Read the model definition and answer for the solid it produces. Units are mm, in the model's axes. A direction names the side the tool comes from. Round coordinates to 2 decimals unless told otherwise and drop trailing zeros. Order: outer loops, then holes, each group sorted by start corner. A loop starts at its lowest first (then second) coordinate and runs counter-clockwise, first axis right, second up. Notation, with made-up numbers: (79, 66) - (91, 66) arc R27 cw to (91, 97) - close; hole circle Ø7 at (47.25, -9.5). An arc over 180 degrees is marked (long way). One line per question, with ' | ' between items. Start each with the question number.
1) For faces 4 (the flat face through (-39, 2, -10)), 5 (the flat face through (44.24, 1.97, 3.73)), determine the directions among +Z, -Z, +X, -X, +Y, -Y from which every point of the face is accessible in a straight line to the end or side of a thin tool.
2) The mould has two halves that part along X. Classify faces 1 (the cylindrical face through (63.733, 1.972, -11.102)), 2 (the flat face through (20, 2, 0)), 3 (the flat face through (1, 2, -14)): pulls with the +X half, pulls with the -X half, needs draft (parallel to the pull), parting line crosses it, or undercut.
3) The part is cut by section A-A, the plane y = 1.4. Count the separate pieces of the cut face and the enclosed holes in it, plus the area to 3 significant figures.
4) Flat-ended cylindrical pins translate along their axes: pin 1 (2 mm diameter, centred on x = -59.47, z = -10, fed in from +Y); pin 2 (2 mm diameter, centred on x = 43, y = 1.5, fed in from +Z); pin 3 (1.5 mm diameter, centred on y = 1, z = -4, fed in from -X). Find the tip coordinate at first contact, or state that the pin passes through.
5) Straight lines are drawn through the part: line 1 (Z direction, x = -4.5, y = 3.45); line 2 (X direction, y = 2.9, z = -8.5); line 3 (X direction, y = 2.75, z = 2). For each, find the intervals that lie inside material, in ascending order. Write a range as from..to.
6) The part is cut by section C-C, the plane z = -0.5. Give the vertices of the cut face in (x, y).
7) The part is cut by section B-B, the plane x = -38. Give the vertices of the cut face in (y, z).
from build123d import *

# Parameters (mm, degrees)
SKETCH_1_R          = 1.5
SKETCH_1_W          = 40
SKETCH_1_H          = 20
EXTRUDE_1_DEPTH     = 4
FILLET_1_R          = 3
FILLET_2_R          = 3
SKETCH_2_R          = 1.75
CUT_EXTRUDE_1_DEPTH = 67.130086355


with BuildPart() as part:
    # 草图1 → 凸台-拉伸1 (new body)
    with BuildSketch(Plane(origin=(0, 0, 0), x_dir=(1, 0, 0), z_dir=(0, 1, 0))):
        with BuildLine():
            Line((-27, -14), (27, -14))
            Line((27, -14), (61.972111671, 6.837249964))
            ThreePointArc((61.972111671, 6.837249964), (63.714640377, 11.169883003), (60, 14))
            Line((60, 14), (27, 14))
            Line((27, 14), (-27, 14))
            Line((-27, 14), (-60, 14))
            ThreePointArc((-60, 14), (-63.714640377, 11.169883003), (-61.972111671, 6.837249964))
            Line((-61.972111671, 6.837249964), (-27, -14))
        make_face()
        with Locations(Location((-23.680960464, 5.529497849, 0), (0, 0, 270))):
            Circle(SKETCH_1_R, mode=Mode.SUBTRACT)
        with Locations(Location((-23.680960464, -5.529497849, 0), (0, 0, 90))):
            Circle(SKETCH_1_R, mode=Mode.SUBTRACT)
        with Locations(Location((23.680960464, -5.529497849, 0), (0, 0, 270))):
            Circle(SKETCH_1_R, mode=Mode.SUBTRACT)
        with Locations(Location((23.680960464, 5.529497849, 0), (0, 0, 90))):
            Circle(SKETCH_1_R, mode=Mode.SUBTRACT)
        Rectangle(SKETCH_1_W, SKETCH_1_H, mode=Mode.SUBTRACT)
        Polygon((30, 10), (59.465601315, 10), (30, -7.556334765), align=None, mode=Mode.SUBTRACT)
        Polygon((-59.465601315, 10), (-30, -7.556334765), (-30, 10), align=None, mode=Mode.SUBTRACT)
    extrude(amount=EXTRUDE_1_DEPTH)

    # 圆角1
    fillet_1_edges = [part.edges().sort_by_distance(p)[0] for p in [
        (59.465601315, 2, -10),
    ]]
    fillet(fillet_1_edges, radius=FILLET_1_R)

    # 圆角2
    fillet_2_edges = [part.edges().sort_by_distance(p)[0] for p in [
        (-59.465601315, 2, -10),
    ]]
    fillet(fillet_2_edges, radius=FILLET_2_R)

    # 草图2 → 切除-拉伸1 (cut, through all)
    with BuildSketch(Plane(origin=(0, 10, 0), x_dir=(1, 0, 0), z_dir=(0, 1, 0))):
        with Locations(Location((-59.465601315, 10, 0), (0, 0, 270))):
            Circle(SKETCH_2_R)
        with Locations(Location((59.465601315, 10, 0), (0, 0, 270))):
            Circle(SKETCH_2_R)
    extrude(amount=-CUT_EXTRUDE_1_DEPTH, mode=Mode.SUBTRACT)


solid = part.part
Values:
1) face 4: +Y, -Y | face 5: +Z, +X, +Y, -Y
2) face 1: pulls with the +X half | face 2: undercut | face 3: needs draft
3) separate pieces: 1 | enclosed holes: 9 | area: 1,440 mm^2
4) pin 1: passes through | pin 2: stops at z = 5.06 | pin 3: stops at x = -58.47
5) line 1: z = -14..-10, 10..14 | line 2: x = -63.48..-60.37, -58.56..-51.17, -30..-20, 20..30, 51.17..58.56, 60.37..63.48 | line 3: x = -47.14..-39.33, -30..-20, 20..30, 39.33..47.14
6) outline: (-51.34, 0) - (-43.52, 0) - (-43.52, 4) - (-51.34, 4) - close; (-30, 0) - (-20, 0) - (-20, 4) - (-30, 4) - close; (20, 0) - (30, 0) - (30, 4) - (20, 4) - close; (43.52, 0) - (51.34, 0) - (51.34, 4) - (43.52, 4) - close
7) outline: (0, -14) - (4, -14) - (4, -10) - (0, -10) - close; (0, 2.79) - (4, 2.79) - (4, 7.45) - (0, 7.45) - close
